For this review, take the finished solid that the model builds, in its own axes (mm). A direction names the side the tool comes from. Coordinates: 2 decimals unless noted, no trailing zeros. Write each loop counter-clockwise with the first axis right and the second up, starting at its lowest first coordinate (ties: lowest second). Pieces come first, ordered by that corner, then holes. Notation, with made-up numbers: M 6,85.25 L 30,85.25 A5 cw 30,92.25 Z; hole C 32,65 d8. An arc over 180 degrees is marked long. Return JSON: item names as keys, results as strings.
```python
from build123d import *

# Parameters (mm, degrees)
SKETCH3_R           = 10.16
CUT_EXTRUDE1_DEPTH  = 2.54
SKETCH5_R           = 4.7625
CUT_EXTRUDE2_DEPTH  = 6.35
SKETCH6_R           = 13.335
SKETCH6_R_2         = 9.525
BOSS_EXTRUDE1_DEPTH = 6.35
SKETCH7_R           = 1.27
CUT_EXTRUDE3_DEPTH  = 25.4
CUT_EXTRUDE4_DEPTH  = 6.35
CUT_EXTRUDE5_DEPTH  = 2.54
SKETCH11_R          = 0.889
CUT_EXTRUDE6_DEPTH  = 55.372


with BuildPart() as part:
    # Sketch2 → Revolve1 (revolve)
    with BuildSketch(Plane(origin=(0, 0, 0), x_dir=(0, 0, -1), z_dir=(1, 0, 0))):
        Polygon((-6.35, 42.32529), (0, 42.32529), (0, 47.625), (2.54, 47.625), (2.54, 0), (0, 0), (0, 39.839805153), (-8.89, 39.839805153), (-8.89, 47.625), (-6.35, 47.625), align=None)
    revolve(axis=Axis((0, 0, 0), (0, 0, -1)))

    # Sketch3 → Cut-Extrude1 (cut)
    with BuildSketch(Plane.XY):
        Circle(SKETCH3_R)
    extrude(amount=-CUT_EXTRUDE1_DEPTH, mode=Mode.SUBTRACT)

    # Sketch4 → Revolve2 (revolve)
    with BuildSketch(Plane(origin=(0, 0, 0), x_dir=(1, 0, 0), z_dir=(0, 1, 0))):
        Polygon((0, 14.2494), (-3.175, 14.2494), (-3.175, 3.175), (-10.16, 3.175), (-10.16, 0), (-13.335, 0), (-13.335, 15.2019), (0, 15.2019), align=None)
    revolve(axis=Axis((0, 0, 0), (0, 0, -1)))

    # Sketch5 → Cut-Extrude2 (cut)
    with BuildSketch(Plane.XY):
        with Locations((0, 22.225)):
            Circle(SKETCH5_R)
    extrude(amount=-CUT_EXTRUDE2_DEPTH, mode=Mode.SUBTRACT)

    # Sketch6 → Boss-Extrude1 (add)
    with BuildSketch(Plane(origin=(0, 0, -15.2019), x_dir=(-1, 0, 0), z_dir=(0, 0, -1))):
        Circle(SKETCH6_R)
        Circle(SKETCH6_R_2, mode=Mode.SUBTRACT)
    extrude(amount=BOSS_EXTRUDE1_DEPTH)

    # Sketch7 → Cut-Extrude3 (cut)
    with BuildSketch(Plane(origin=(0, 0, 0), x_dir=(0, 0, -1), z_dir=(1, 0, 0))):
        with Locations((8.962319715, 0)):
            Circle(SKETCH7_R)
    extrude(amount=-CUT_EXTRUDE3_DEPTH, mode=Mode.SUBTRACT)

    # Sketch8 → Cut-Extrude4 (cut)
    with BuildSketch(Plane(origin=(0, 0, -21.5519), x_dir=(-1, 0, 0), z_dir=(0, 0, -1))):
        with BuildLine():
            Line((2.725322184, 6.579509779), (5.964417729, 14.399378174))
            ThreePointArc((5.964417729, 14.399378174), (0, 15.585774625), (-5.964417729, 14.399378174))
            Line((-5.964417729, 14.399378174), (-2.725322184, 6.579509779))
            ThreePointArc((-2.725322184, 6.579509779), (0, 7.121610066), (2.725322184, 6.579509779))
        make_face()
    extrude(amount=-CUT_EXTRUDE4_DEPTH, mode=Mode.SUBTRACT)

    # Sketch10 → Cut-Extrude5 (cut)
    with BuildSketch(Plane(origin=(0, 0, -19.0119), x_dir=(-1, 0, 0), z_dir=(0, 0, -1))):
        with BuildLine():
            Line((6.29135007, 1.685762171), (16.396038566, 4.393305293))
            ThreePointArc((16.396038566, 4.393305293), (14.700286019, 8.48721409), (12.002733273, 12.002733273))
            Line((12.002733273, 12.002733273), (4.6055879, 4.6055879))
            ThreePointArc((4.6055879, 4.6055879), (5.64067016, 3.256642435), (6.29135007, 1.685762171))
        make_face()
        with BuildLine():
            Line((-4.6055879, 4.6055879), (-12.002733273, 12.002733273))
            ThreePointArc((-12.002733273, 12.002733273), (-14.700286019, 8.48721409), (-16.396038566, 4.393305293))
            Line((-16.396038566, 4.393305293), (-6.29135007, 1.685762171))
            ThreePointArc((-6.29135007, 1.685762171), (-5.64067016, 3.256642435), (-4.6055879, 4.6055879))
        make_face()
    extrude(amount=-CUT_EXTRUDE5_DEPTH, mode=Mode.SUBTRACT)

    # Sketch11 → Cut-Extrude6 (cut)
    with BuildSketch(Plane(origin=(0, 0, 0), x_dir=(1, 0, 0), z_dir=(0, 1, 0))):
        with Locations((0, -3.870418615)):
            Circle(SKETCH11_R)
    extrude(amount=CUT_EXTRUDE6_DEPTH, mode=Mode.SUBTRACT)


solid = part.part
```
1. Wall thickness on L1, parallel to X at y = 0, z = -17 (3 decimals); L2, parallel to Z at x = 20.5, y = 40; L3, parallel to X at y = 0, z = -1.45 (3 decimals): over which ranges is each line inside the solid? List them lowest first. Write a range as from..to.
Checks:
{"L1": "-13.335..-9.525, 9.525..13.335", "L2": "-2.54..0, 6.35..8.89", "L3": "-47.625..-10.16, 10.16..47.625"}
2. For faces 5 (the face through (12.71, 40.37, 3.13)), 6 (the face through (-8, 8, -18)), 7 (the face through (-4.364, 10.535, -18.421)), 8 (the face through (-8, -8, 0)), list the 3-axis set-ups (+Z, -Z, +X, -X, +Y, -Y) from which the entire face can be reached by the end or side of a thin tool; tool diameter is ignored.
Checks:
{"face 5": "none", "face 6": "-X", "face 7": "-Z, +Y", "face 8": "+Z"}
3. We need section A-A (x = 14.5). State the section outline as (y, z) points.
Checks:
{"outline": "M -45.36,-2.54 L 45.36,-2.54 L 45.36,0 L 39.76,0 L 39.76,6.35 L 45.36,6.35 L 45.36,8.89 L 37.11,8.89 L 37.11,0 L -37.11,0 L -37.11,8.89 L -45.36,8.89 L -45.36,6.35 L -39.76,6.35 L -39.76,0 L -45.36,0 Z"}
4. We need section C-C (x = -41). State the section outline as (y, z) points, plus the area to 3 significant figures.
Checks:
{"outline": "M -24.23,-2.54 L 24.23,-2.54 L 24.23,0 L 10.51,0 L 10.51,6.35 L 24.23,6.35 L 24.23,8.89 L -24.23,8.89 L -24.23,6.35 L -10.51,6.35 L -10.51,0 L -24.23,0 Z", "area": "380 mm2"}
5. We need section B-B (y = -25.5). State the section outline as (x, z) points, plus the area to 3 significant figures.
Checks:
{"outline": "M -40.22,-2.54 L 40.22,-2.54 L 40.22,0 L 33.78,0 L 33.78,6.35 L 40.22,6.35 L 40.22,8.89 L 30.61,8.89 L 30.61,0 L -30.61,0 L -30.61,8.89 L -40.22,8.89 L -40.22,6.35 L -33.78,6.35 L -33.78,0 L -40.22,0 Z", "area": "293 mm2"}
6. Clearance check with flat-ended pins moving along their axes: pin 1 Ø7 at (x, y) = (0.5, -1.5) entering from +Z (3 decimals); pin 2 Ø5.5 at (x, y) = (0, 0) entering from +Z; pin 3 Ø1.5 at (y, z) = (0, -8.96) entering from -X; pin 4 Ø7.5 at (x, y) = (0, 22.225) entering from -Z. State where each tip first meets the part, or that it passes through.
Checks:
{"pin 1": "z = -3.175", "pin 2": "z = -14.25", "pin 3": "x = 3.09", "pin 4": "through"}
7. Draft analysis for pull direction Z (two halves, no side actions). For faces 1 (the face through (-2.4, 2.4, -3.175)), 2 (the face through (3.17, 0.14, -8.63)), 3 (the face through (10, 6, -16.472)), 4 (the face through (-8.049, -0.486, -10.135)), state which applies: +Z half, -Z half, draft (parallel to the pull), parting line (faces both ways), or undercut.
Checks:
{"face 1": "+Z half", "face 2": "draft", "face 3": "undercut", "face 4": "undercut"}
